Autodesk Inventor part; units mm, degrees
ref_plane "YZ Plane" through (0, 0, 0) normal (1, 0, 0) x (0, 1, 0)
ref_plane "XZ Plane" through (0, 0, 0) normal (0, 1, 0) x (-1, 0, 0)
ref_plane "XY Plane" through (0, 0, 0) normal (0, 0, 1) x (1, 0, 0)
sketch "草图1" plane through (0, 0, 0) normal (1, 0, 0) x (0, 1, 0)
  line L0 (9.7546, -15.7991) -> (9.7546, -18.7991)
  line L1 (20.7546, -18.7991) -> (9.7546, -18.7991)
  line L2 (20.7546, -18.7991) -> (20.7546, -10.7991)
  line L3 (18.7546, -8.7991) -> (20.7546, -10.7991)
  line L4 (18.7546, -8.7991) -> (-19.2454, -8.7991)
  line L5 (-21.2454, -10.7991) -> (-19.2454, -8.7991)
  line L6 (-21.2454, -10.7991) -> (-21.2454, -18.7991)
  line L7 (-10.2454, -18.7991) -> (-21.2454, -18.7991)
  line L8 (-10.2454, -18.7991) -> (-10.2454, -15.7991)
  line L9 (-10.2454, -15.7991) -> (-7.2454, -15.7991)
  line L10 (-7.2454, -15.7991) -> (-7.2454, -13.7991)
  line L11 (-7.2454, -13.7991) -> (-10.2454, -13.7991)
  line L12 (-10.2454, -13.7991) -> (-10.2454, -10.7991)
  line L13 (-10.2454, -10.7991) -> (9.7546, -10.7991)
  line L14 (9.7546, -10.7991) -> (9.7546, -13.7991)
  line L15 (9.7546, -13.7991) -> (6.7546, -13.7991)
  line L16 (6.7546, -13.7991) -> (6.7546, -15.7991)
  line L17 (6.7546, -15.7991) -> (9.7546, -15.7991)
  line L18 (9.7546, -18.7991) -> (12.7546, -18.7991)
  line L19 (12.7546, -18.7991) -> (12.7546, -6.7991)
  line L20 (-10.2454, -18.7991) -> (-13.2454, -18.7991)
  line L21 (-13.2454, -18.7991) -> (-13.2454, -6.7991)
  line L22 (-13.2454, -6.7991) -> (12.7546, -6.7991)
  dimension "d0" = 3
  dimension "d1" = 12
extrude "拉伸1" add sketch "草图1" along normal blind 40 contours L17 L16 L15 L14 L13 L12 L11 L10 L9 L8 L7 L21 L4 L19 L1 L0 | L4 L21 L22 L19
sketch "草图2" plane through (0, -13.2454, -6.7991) normal (0, 0, 1) x (1, 0, 0)
  line L0 (40, 26) -> (40, 0)
  line L1 (0, 0) -> (40, 0)
  line L2 (40, 0) -> (40, 8)
  line L3 (40, 8) -> (0, 8)
  line L4 (0, 8) -> (0, 0)
  line L5 (0, 26) -> (40, 26)
  line L6 (0, 26) -> (40, 26)
  line L7 (40, 26) -> (40, 18)
  line L8 (40, 18) -> (0, 18)
  line L9 (0, 18) -> (0, 26)
  point P0 (0, 13.2454)
  dimension "d4" = 8
  dimension "d5" = 8
extrude "拉伸2" add sketch "草图2" along normal blind 2
sketch "草图3" plane through (0, -13.2454, -4.7991) normal (0, 0, 1) x (1, 0, 0)
  line L0 (40, 26) -> (0, 26)
  line L1 (0, 26) -> (0, 18)
  line L2 (40, 18) -> (40, 26)
  line L3 (0, 0) -> (40, 0)
  point P0 (0, 13.2454)
  point P1 (8, 22)
  point P2 (32, 22)
  point P3 (32, 4)
  point P4 (8, 4)
  dimension "d8" = 4
  dimension "d9" = 8
  dimension "d10" = 8
  dimension "d11" = 4
hole "孔1" at (8, 8.7546, -4.7991) at (32, 8.7546, -4.7991) at (32, -9.2454, -4.7991) at (8, -9.2454, -4.7991) direction (0, 0, -1) diameter 3.242 depth 3
properties part number "滑块3"
The listing builds one solid part. Answer for the finished solid, in the listing's coordinates (mm). A direction names the side the tool comes from. Coordinates: 2 decimals unless noted, no trailing zeros. Loops run counter-clockwise (first coordinate to the right, second up) from the corner with the lowest first, then second, coordinate; pieces in that order, holes last.
1) Determine the mould class of faces 1 (the face through (20, 12.755, -12)), 2 (the face through (20, -12, -18.799)), 3 (the face through (32, -9, -7.799)), 4 (the face through (20, -13.245, -12)) for opening direction Y: pulls with the +Y half, pulls with the -Y half, needs draft (parallel to the pull), parting line crosses it, or undercut.
2) Find section B-B on x = 8. Write down the section's boundary in (y, z), then the cut area to 3 significant figures.
3) Find section D-D on x = 28. Write down the section's boundary in (y, z), then the cut area to 3 significant figures.
4) Find section A-A on z = -16.5. Write down the section's boundary in (x, y).
5) A tool of negligible diameter and unlimited length cuts with its end or side. For faces 5 (the face through (20, -9, -13.799)), 6 (the face through (8.621, -10.743, -6.32)), 7 (the face through (20, 4.755, -6)), 8 (the face through (20, 9.755, -17)), from which of +Z, -Z, +X, -X, +Y, -Y can it reach the whole face along a straight path? Write none if from no direction.
6) Find the intervals of material crossed by L1, parallel to X at y = -9.25, z = -7.75; L2, parallel to Y at x = 8, z = -6.6; L3, parallel to Z at x = 28, y = 7.75, in increasing order.
7) Flat-ended cylindrical pins translate along their axes: pin 1 Ø3 at (x, y) = (9.5, -0.5) entering from -Z; pin 2 Ø8 at (x, y) = (32, 5) entering from -Z; pin 3 Ø1 at (x, y) = (7.5, 8.5) entering from +Z; pin 4 Ø2.5 at (x, y) = (7.5, -9.5) entering from +Z. Find the tip coordinate at first contact, or state that the pin passes through.
8) Find section C-C on y = -8.75. Write down the section's boundary in (x, z), then the cut area to 3 significant figures.
Values:
1. face 1: pulls with the +Y half
1. face 2: needs draft
1. face 3: undercut
1. face 4: pulls with the -Y half
2. outline: (-13.25, -18.8) - (-10.25, -18.8) - (-10.25, -15.8) - (-7.25, -15.8) - (-7.25, -13.8) - (-10.25, -13.8) - (-10.25, -10.8) - (9.75, -10.8) - (9.75, -13.8) - (6.75, -13.8) - (6.75, -15.8) - (9.75, -15.8) - (9.75, -18.8) - (12.75, -18.8) - (12.75, -4.8) - (10.38, -4.8) - (10.38, -7.8) - (7.13, -7.8) - (7.13, -4.8) - (4.75, -4.8) - (4.75, -6.8) - (-5.25, -6.8) - (-5.25, -4.8) - (-7.62, -4.8) - (-7.62, -7.8) - (-10.87, -7.8) - (-10.87, -4.8) - (-13.25, -4.8) - close
2. area: 177 mm2
3. outline: (-13.25, -18.8) - (-10.25, -18.8) - (-10.25, -15.8) - (-7.25, -15.8) - (-7.25, -13.8) - (-10.25, -13.8) - (-10.25, -10.8) - (9.75, -10.8) - (9.75, -13.8) - (6.75, -13.8) - (6.75, -15.8) - (9.75, -15.8) - (9.75, -18.8) - (12.75, -18.8) - (12.75, -4.8) - (4.75, -4.8) - (4.75, -6.8) - (-5.25, -6.8) - (-5.25, -4.8) - (-13.25, -4.8) - close
3. area: 196 mm2
4. outline: (0, -13.25) - (40, -13.25) - (40, -10.25) - (0, -10.25) - close; (0, 9.75) - (40, 9.75) - (40, 12.75) - (0, 12.75) - close
5. face 5: +X, -X
5. face 6: +Z
5. face 7: +Z, +X, -X
5. face 8: -Z, +X, -X
6. L1: x = 0 to 6.38, 9.62 to 30.38, 33.62 to 40
6. L2: y = -13.25 to -10.87, -7.62 to -5.25, 4.75 to 7.13, 10.38 to 12.75
6. L3: z = -15.8 to -13.8, -10.8 to -4.8
7. pin 1: stops at z = -10.8
7. pin 2: stops at z = -15.8
7. pin 3: stops at z = -7.8
7. pin 4: stops at z = -4.8
8. outline: (0, -15.8) - (40, -15.8) - (40, -13.8) - (0, -13.8) - close; (0, -10.8) - (40, -10.8) - (40, -4.8) - (33.54, -4.8) - (33.54, -7.8) - (30.46, -7.8) - (30.46, -4.8) - (9.54, -4.8) - (9.54, -7.8) - (6.46, -7.8) - (6.46, -4.8) - (0, -4.8) - close
8. area: 301 mm2
